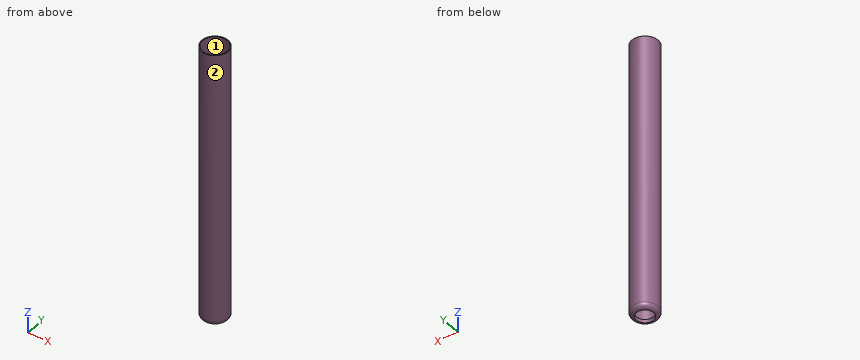
from build123d import *

# Parameters (mm, degrees)
SKETCH1_R           = 14.5
BOSS_EXTRUDE1_DEPTH = 304.8
SKETCH2_R           = 13.5
CUT_EXTRUDE1_DEPTH  = 301
FILLET2_R           = 5
SKETCH8_R           = 9.5
CUT_EXTRUDE2_DEPTH  = 10


with BuildPart() as part:
    # Sketch1 → Boss-Extrude1 (new body)
    with BuildSketch(Plane.XY):
        Circle(SKETCH1_R)
    extrude(amount=-BOSS_EXTRUDE1_DEPTH)

    # Sketch2 → Cut-Extrude1 (cut)
    with BuildSketch(Plane.XY):
        Circle(SKETCH2_R)
    extrude(amount=-CUT_EXTRUDE1_DEPTH, mode=Mode.SUBTRACT)

    # Fillet2
    fillet2_edges = [part.edges().sort_by_distance(p)[0] for p in [
        (-14.5, 0, -304.8),
    ]]
    fillet(fillet2_edges, radius=FILLET2_R)

    # Sketch8 → Cut-Extrude2 (cut)
    with BuildSketch(Plane(origin=(0, 0, -304.8), x_dir=(-1, 0, 0), z_dir=(0, 0, -1))):
        with Locations(Location((0, 0, 0), (0, 0, 180))):
            Circle(SKETCH8_R)
    extrude(amount=-CUT_EXTRUDE2_DEPTH, mode=Mode.SUBTRACT)


solid = part.part
Input: part model. Units: mm. Frame: model coordinates. Face numbers are marked on the shaded views. Coordinates: 2 decimals unless noted, no trailing zeros. Loops run counter-clockwise (first coordinate to the right, second up) from the corner with the lowest first, then second, coordinate; pieces in that order, holes last.
Q1. Material intervals for line 1 (Y direction, x = 0, z = -111.5); line 2 (Z direction, x = -1.25, y = 10); line 3 (Y direction, x = 4.75, z = -215), sorted ascending.
Q2. Cut plane C-C (z = -286). Output: boundary loops of the cut face in (x, y).
Q3. Contact query for flat-ended pins moving along their axis: pin 1 (3 mm diameter, centred on y = 5.5, z = -188, fed in from -X); pin 2 (5 mm diameter, centred on x = -6, z = -208.5, fed in from +Y); pin 3 (8 mm diameter, centred on x = -9, z = -102.5, fed in from -Y). Output: stop coordinate, or through.
Q4. Cut plane A-A (y = 0). Output: boundary loops of the cut face in (x, z).
Q5. Draft query along X for the marked faces 1 and 2. Return one class per face: +X half, -X half, draft (parallel to the pull), parting line (faces both ways), or undercut.
Working result:
1. line 1: y = -14.5 to -13.5, 13.5 to 14.5
1. line 2: z = -304.77 to -301
1. line 3: y = -13.7 to -12.64, 12.64 to 13.7
2. outline: circle Ø29 at (0, 0); hole circle Ø27 at (0, 0)
3. pin 1: stops at x = -13.94
3. pin 2: stops at y = 14.07
3. pin 3: stops at y = -13.61
4. outline: (-14.5, -299.8) arc R5 ccw to (-9.5, -304.8) - (-9.5, -301) - (-13.5, -301) - (-13.5, 0) - (-14.5, 0) - close; (9.5, -304.8) arc R5 ccw to (14.5, -299.8) - (14.5, 0) - (13.5, 0) - (13.5, -301) - (9.5, -301) - close
5. face 1: undercut
5. face 2: parting line
